```python
from build123d import *

# Parameters (mm, degrees)
SKETCH003_R        = 34.629948
PAD001_DEPTH       = 10
SKETCH004_R        = 21.305657
POCKET_DEPTH       = 5
SKETCH005_R        = 7.329797
POCKET001_DEPTH    = 11
POCKET002_DEPTH    = 38
POLARPATTERN_COUNT = 22


with BuildPart() as part:
    # Sketch003 → Pad001 (new body)
    with BuildSketch(Plane.XY):
        Circle(SKETCH003_R)
    extrude(amount=PAD001_DEPTH)

    # Sketch004 → Pocket (cut)
    with BuildSketch(Plane.XY):
        Circle(SKETCH004_R)
    extrude(amount=POCKET_DEPTH, mode=Mode.SUBTRACT)

    # Sketch005 → Pocket001 (cut)
    with BuildSketch(Plane.XY):
        Circle(SKETCH005_R)
    extrude(amount=POCKET001_DEPTH, mode=Mode.SUBTRACT)

    # Sketch006 → Pocket002 (cut)
    with BuildSketch(Plane.YZ):
        Polygon((0, 0), (2.410471, 4.960438), (5.179447, 0), align=None)
    pocket002 = extrude(amount=-POCKET002_DEPTH, mode=Mode.SUBTRACT)

    # PolarPattern: Pocket002 ×22 about axis
    polarpattern_axis = Axis((0, 0, 0), (0, 0, 1))
    for i in range(1, POLARPATTERN_COUNT):
        add(pocket002.rotate(polarpattern_axis, i * 360 / POLARPATTERN_COUNT), mode=Mode.SUBTRACT)


solid = part.part
```
Input: part model. Units: mm. Frame: model coordinates. A direction names the side the tool comes from. Round coordinates to 2 decimals unless told otherwise and drop trailing zeros. One line per item, written item: value. Start each with the question number.
(1) Contact query for flat-ended pins moving along their axis: P1, Ø6, axis at x = 24.5, z = 6, coming from the +Y side; P2, Ø19, axis at x = 0, y = 0, coming from the +Z side; P3, Ø1.5, axis at y = -19, z = 7, coming from the -X side; P4, Ø3, axis at y = 11, z = 7, coming from the +X side. Output: stop coordinate, or through.
(2) Draft query along Y for faces 3 (the flat face through (12.632, 24.799, 2.445)), 4 (the flat face through (-18, -23, 0)). Return one class per face: +Y half, -Y half, draft (parallel to the pull), parting line (faces both ways), or undercut.
(3) Access query for faces 1 (the cylindrical face through (-15.7, 14.4, 3.6)), 2 (the flat face through (-6, 29, 0)). Directions: +Z, -Z, +X, -X, +Y, -Y. A direction counts if a zero-diameter tool reaches every point of the face in a straight line with its end or side. Return the directions, or none.
(4) Ray query, line 1 (Y direction, x = -7.5, z = 4.75); line 2 (X direction, y = -15.5, z = 0.5); line 3 (X direction, y = -16.5, z = 3.5). Return the intervals inside material, ascending. Write a range as [from, to].
(5) Section A-A, the plane z = 3.5. Count the separate pieces of the cut face and the enclosed holes in it, plus the area to 3 significant figures.
Results below:
1. P1: y = 27.15
1. P2: z = 10
1. P3: x = -29.43
1. P4: x = 33.3
2. face 3: undercut
2. face 4: draft
3. face 1: -Z
3. face 2: -Z, +X, -X, +Y, -Y
4. line 1: [-33.81, -19.94], [19.94, 21.98], [22.51, 33.81]
4. line 2: [-24.57, -19.91], [14.62, 15.05], [23.67, 30.97]
4. line 3: [-28.82, -18.57], [-16.55, -13.48], [13.48, 19.71], [22.53, 30.45]
5. separate pieces: 22
5. enclosed holes: 0
5. area: 1,890 mm^2
